Could you check a few things on this drawing? It's one solid part, dimensions in mm from its lowest x, y, z. Coordinates: 2 decimals unless noted, no trailing zeros. Write each loop counter-clockwise with the first axis right and the second up, starting at its lowest first coordinate (ties: lowest second). Pieces come first, ordered by that corner, then holes. Notation, with made-up numbers: (-24.75, 80.5) - (18.25, 80.5) arc R20 ccw to (18.25, 95.5) - close; hole circle Ø10 at (-38.5, 62.25). An arc over 180 degrees is marked (long way). Answer as a JSON object with one key per item and string values. Group by question number.
1) Will these pins go through, and if not, where does the flat tip stop? pin 1 Ø17 at (y, z) = (152.4, 22.225) entering from +X; pin 2 Ø1.5 at (x, y) = (2.5, 67.5) entering from -Z.
2) Please list where these lines run through material, in increasing order: line 1 along Z through (x, y) = (4.5, 165.1) (3 decimals); line 2 along Y through (x, z) = (2.25, 137); line 3 along Y through (x, z) = (6, 87).
3) If we section it at B-B (z = 104): Write out the boundary of the cut face in (x, y), plus the area to 3 significant figures.
4) If we section it at C-C (x = 1.75): State how many separate pieces and enclosed holes the cut face has, plus the area to 3 significant figures.
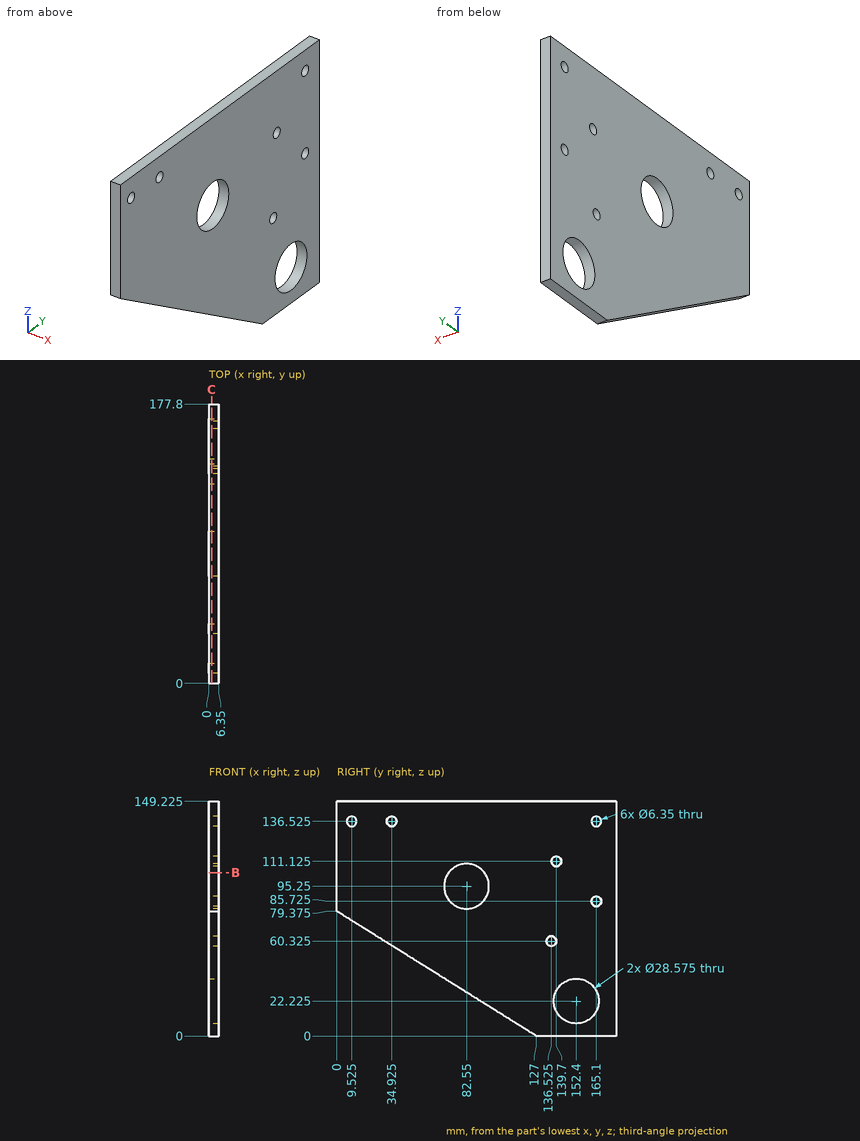
Here are the results:
{
 "1": {"pin 1": "passes through", "pin 2": "stops at z = 36.72"},
 "2": {"line 1": "z = 0 to 15.68, 28.77 to 82.55, 88.9 to 133.35, 139.7 to 149.225", "line 2": "y = 0 to 6.39, 12.66 to 31.79, 38.06 to 161.96, 168.24 to 177.8", "line 3": "y = 0 to 70.89, 94.21 to 162.19, 168.01 to 177.8"},
 "3": {"outline": "(0, 0) - (6.35, 0) - (6.35, 71.26) - (0, 71.26) - close; (0, 93.84) - (6.35, 93.84) - (6.35, 177.8) - (0, 177.8) - close", "area": "986 mm²"},
 "4": {"separate pieces": "1", "enclosed holes": "8", "area": "20,000 mm²"}
}
